from build123d import *

# Parameters (mm, degrees)
F0_W           = 3.35
F0_H           = 5
F1_DEPTH       = 12
F3_D           = 4
F3_DEPTH       = 25
F3_CBORE_D     = 10
F3_CBORE_DEPTH = 4
F3_TIP         = 1.2017212381
F5_D           = 4
F5_DEPTH       = 25
F5_TIP         = 1.2017212381
F6_DEPTH       = 2
F7_T1_DEPTH    = 17
F7_T3_DEPTH    = 85


# Not quite as in the source:
# - a fillet or chamfer that OpenCascade refuses, or shapes differently, is made with other operations: its cross-section is extruded or revolved along the edge and cut away or added


with BuildPart() as f1:
    # F0 (on Front) → F1 (new body)
    with BuildSketch(Plane.XZ):
        with Locations((8.425, 2.5)):
            Rectangle(F0_W, F0_H)
        with Locations((11.775, 2.5)):
            Rectangle(F0_W, F0_H)
        Polygon((0, 5), (6.75, 5), (10.1, 5), (10.1, 12), (0, 12), align=None)
        Polygon((10.1, 12), (10.1, 5), (13.45, 5), (66.55, 5), (69.9, 5), (69.9, 12), align=None)
        with Locations((68.225, 2.5)):
            Rectangle(F0_W, F0_H)
        Polygon((80, 12), (69.9, 12), (69.9, 5), (73.25, 5), (80, 5), align=None)
        with Locations((71.575, 2.5)):
            Rectangle(F0_W, F0_H)
    extrude(amount=F1_DEPTH)

    # F3
    with Locations(Plane.XY.offset(12)):
        with Locations((10.1, -6), (69.9, -6)):
            CounterBoreHole(F3_D / 2, F3_CBORE_D / 2, F3_CBORE_DEPTH, depth=F3_DEPTH)
            with Locations((0, 0, -(F3_DEPTH + F3_TIP / 2))):  # 118° drill point
                Cone(0, F3_D / 2, F3_TIP, mode=Mode.SUBTRACT)

    # F5
    with Locations(Plane.XZ.offset(12)):
        with Locations((40, 8.5)):
            Hole(F5_D / 2, depth=F5_DEPTH)
            with Locations((0, 0, -(F5_DEPTH + F5_TIP / 2))):  # 118° drill point
                Cone(0, F5_D / 2, F5_TIP, mode=Mode.SUBTRACT)

    # F4 (on face) → F6 (cut)
    with BuildSketch(Plane.XZ.offset(12)):
        with BuildLine():
            Line((38.0252040749, 11.9131824428), (36.0587919372, 8.5))
            Line((36.0587919372, 8.5), (38.5835167795, 8.5))
            ThreePointArc((38.5835167795, 8.5), (38.9983951094, 9.5016048906), (40, 9.9164832205))
            Line((40, 9.9164832205), (40, 11.9150014487))
            Line((40, 11.9150014487), (38.0252040749, 11.9131824428))
        make_face()
        with BuildLine():
            Line((38.5835167795, 8.5), (36.0587919372, 8.5))
            Line((36.0587919372, 8.5), (36.0566993343, 8.496367783))
            Line((36.0566993343, 8.496367783), (38.0314952594, 5.0831853402))
            Line((38.0314952594, 5.0831853402), (40, 5.0849985513))
            Line((40, 5.0849985513), (40, 7.0835167795))
            ThreePointArc((40, 7.0835167795), (38.9983951094, 7.4983951094), (38.5835167795, 8.5))
        make_face()
        with BuildLine():
            Line((40, 11.9150014487), (40, 9.9164832205))
            ThreePointArc((40, 9.9164832205), (41.0016048906, 9.5016048906), (41.4164832205, 8.5))
            Line((41.4164832205, 8.5), (43.9412080628, 8.5))
            Line((43.9412080628, 8.5), (43.9433006657, 8.503632217))
            Line((43.9433006657, 8.503632217), (41.9685047406, 11.9168146598))
            Line((41.9685047406, 11.9168146598), (40, 11.9150014487))
        make_face()
        with BuildLine():
            ThreePointArc((41.4164832205, 8.5), (41.0016048906, 7.4983951094), (40, 7.0835167795))
            Line((40, 7.0835167795), (40, 5.0849985513))
            Line((40, 5.0849985513), (41.9747959251, 5.0868175572))
            Line((41.9747959251, 5.0868175572), (43.9412080628, 8.5))
            Line((43.9412080628, 8.5), (41.4164832205, 8.5))
        make_face()
    extrude(amount=-F6_DEPTH, mode=Mode.SUBTRACT)

    # F7: fillet of radius 1 on 6 edges, made by hand

    # F7_s2 → F7_t1 (cut)
    with BuildSketch(Plane.XZ.offset(-2.5)):
        with BuildLine():
            ThreePointArc((79, 12), (79.7071067812, 11.7071067812), (80, 11))
            Line((80, 11), (80, 12))
            Line((80, 12), (79, 12))
        make_face()
        with BuildLine():
            ThreePointArc((0, 11), (0.2928932188, 11.7071067812), (1, 12))
            Line((1, 12), (0, 12))
            Line((0, 12), (0, 11))
        make_face()
    extrude(amount=F7_T1_DEPTH, mode=Mode.SUBTRACT)

    # F7_s4 → F7_t3 (cut)
    with BuildSketch(Plane.YZ.offset(-2.5)):
        with BuildLine():
            ThreePointArc((0, 11), (-0.2928932188, 11.7071067812), (-1, 12))
            Line((-1, 12), (0, 12))
            Line((0, 12), (0, 11))
        make_face()
        with BuildLine():
            ThreePointArc((-12, 11), (-11.7071067812, 11.7071067812), (-11, 12))
            Line((-11, 12), (-12, 12))
            Line((-12, 12), (-12, 11))
        make_face()
    extrude(amount=F7_T3_DEPTH, mode=Mode.SUBTRACT)

    # F7_s5 → F7_t6 (revolve, cut)
    with BuildSketch(Plane.XZ.offset(6)):
        with BuildLine():
            ThreePointArc((75.9, 12), (75.1928932188, 11.7071067812), (74.9, 11))
            Line((74.9, 11), (74.9, 12))
            Line((74.9, 12), (75.9, 12))
        make_face()
    revolve(axis=Axis((69.9, -6, 12), (0, 0, 1)), mode=Mode.SUBTRACT)

    # F7_s7 → F7_t8 (revolve, cut)
    with BuildSketch(Plane.XZ.offset(6)):
        with BuildLine():
            ThreePointArc((16.1, 12), (15.3928932188, 11.7071067812), (15.1, 11))
            Line((15.1, 11), (15.1, 12))
            Line((15.1, 12), (16.1, 12))
        make_face()
    revolve(axis=Axis((10.1, -6, 12), (0, 0, 1)), mode=Mode.SUBTRACT)


solid = f1.part
Source: CAD feature listing. Evaluate the final solid. Frame: model axes, mm. A direction names the side the tool comes from. Give positions to 0.01 mm unless a question says otherwise; leave off trailing zeros. Write each loop counter-clockwise with the first axis right and the second up, starting at its lowest first coordinate (ties: lowest second). Pieces come first, ordered by that corner, then holes. Notation, with made-up numbers: M 36,-7 L 51,-7 A13 cw 51,8 Z; hole C -34.75,50 d2. An arc over 180 degrees is marked long. Return JSON: item names as keys, results as strings. Group by question number.
1) Draft query along Z for faces 1 (the face through (41.474, -4.93, 9.852)), 2 (the face through (40, -6, 5)), 3 (the face through (6.75, -6, 2)). Return one class per face: released by +Z, released by -Z, zero draft, split by the parting line, or undercut.
2) Cut plane C-C, the plane z = 5.75. Output: boundary loops of the cut face in (x, y).
3) Set-up query: faces 4 (the face through (3, -6, 5)), 5 (the face through (13.45, -6, 2)), 6 (the face through (37.03, -11.014, 6.814)), 7 (the face through (6.1, -9, 9.5)), 8 (the face through (73.25, -6, 2)). Return all of +Z, -Z, +X, -X, +Y, -Y with unobstructed straight access to the full face (end or side cutting, diameter ignored); none if empty.
4) Cut plane B-B, the plane x = 51.5. Output: boundary loops of the cut face in (y, z), then the cut area to 3 significant figures.
5) First-contact query: pin 1 Ø2.5 at (y, z) = (-6.5, 3) entering from -X; pin 2 Ø3 at (y, z) = (-3, 4.5) entering from -X; pin 3 Ø1.5 at (y, z) = (-6, 1.5) entering from +X; pin 4 Ø3 at (x, y) = (70.5, -6.5) entering from +Z. Flat tips, straight axial feed; report the tip coordinate or a pass-through.
6) Ray query, L1, parallel to X at y = -11, z = 2; L2, parallel to Y at x = 69.9, z = 10.1; L3, parallel to X at y = -10.5, z = 9. Return the intervals inside material, ascending.
7) Cut plane A-A, the plane y = -6. Give the number of separate pieces and of enclosed holes in the cut face, then the cut area to 3 significant figures.
8) Cut plane D-D, the plane x = 10.1. Output: boundary loops of the cut face in (y, z), then the cut area to 3 significant figures.
Data:
{
 "1": {"face 1": "undercut", "face 2": "released by -Z", "face 3": "zero draft"},
 "2": {"outline": "M 0,-12 L 37.65,-12 L 37.65,-10 L 42.36,-10 L 42.36,-12 L 80,-12 L 80,0 L 0,0 Z; hole C 10.1,-6 d4; hole C 69.9,-6 d4"},
 "3": {"face 4": "-Z, -X, +Y, -Y", "face 5": "-Z, +Y, -Y", "face 6": "-Y", "face 7": "+Z", "face 8": "-Z, +X, +Y, -Y"},
 "4": {"outline": "M -12,5 L 0,5 L 0,11 A1 ccw -1,12 L -11,12 A1 ccw -12,11 Z", "area": "83.6 mm²"},
 "5": {"pin 1": "stops at x = 6.75", "pin 2": "stops at x = 0", "pin 3": "stops at x = 73.25", "pin 4": "stops at z = 8"},
 "6": {"L1": "x = 6.75 to 13.45, 66.55 to 73.25", "L2": "y = -12 to -11, -1 to 0", "L3": "x = 0 to 7.92, 12.28 to 36.35, 43.66 to 67.72, 72.08 to 80"},
 "7": {"separate pieces": "3", "enclosed holes": "1", "area": "469 mm²"},
 "8": {"outline": "M -12,0 L -8,0 L -8,8 L -11,8 L -11,11 A1 ccw -11.5,11.87 A1 ccw -12,11 Z; M -4,0 L 0,0 L 0,11 A1 ccw -0.5,11.87 A1 ccw -1,11 L -1,8 L -4,8 Z", "area": "71.2 mm²"}
}
